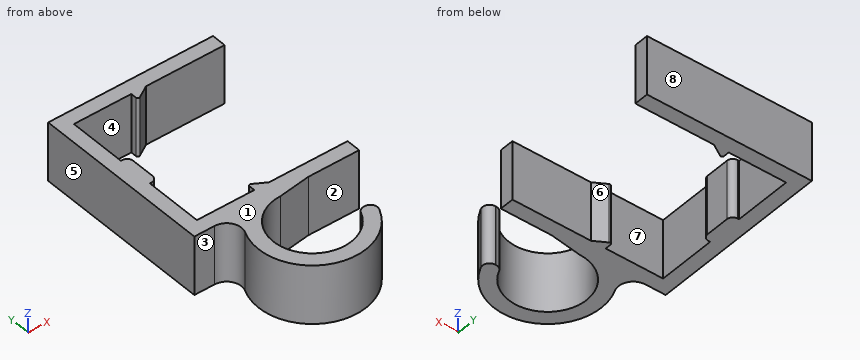
from build123d import *

# Parameters (mm, degrees)
F0_W     = 1.25
F0_H     = 6
F1_DEPTH = 10
F3_DEPTH = 10
F4_R     = 1.2
F5_R     = 2.5
F6_R     = 1
F7_R     = 0.3


with BuildPart() as f1:
    # F0 (on Top) → F1 (new body)
    with BuildSketch(Plane.XY):
        Polygon((0, -2.4), (0, 0), (-28, 0), (-28, -30.3), (0, -30.3), (0, -27.9), (-13.35, -27.9), (-15.85, -27.9), (-25.6, -27.9), (-25.6, -18.15), (-25.6, -12.15), (-25.6, -2.4), (-15.85, -2.4), (-13.35, -2.4), align=None)
        Polygon((-15.85, -3.9), (-13.35, -2.4), (-15.85, -2.4), align=None)
        Polygon((-15.85, -27.9), (-13.35, -27.9), (-15.85, -26.4), align=None)
        with Locations((-24.975, -15.15)):
            Rectangle(F0_W, F0_H)
    extrude(amount=F1_DEPTH)

    # F2 (on face) → F3 (join)
    with BuildSketch(Plane.XY.offset(10)):
        with BuildLine():
            ThreePointArc((-7.6731015896, -39.6488182922), (-19.3342450038, -41.6128057076), (-14, -31.0588802515))
            Line((-14, -31.0588802515), (-8.6386627198, -30.3))
            ThreePointArc((-8.6386627198, -30.3), (-22.5307966917, -40.9228820738), (-5.0890716816, -39.6488182922))
            Line((-5.0890716816, -39.6488182922), (-7.6731015896, -39.6488182922))
        make_face()
    extrude(amount=-F3_DEPTH)

    # F4
    f4_edges = [f1.edges().sort_by_distance(p)[0] for p in [
        (-7.673102, -39.648818, 5),
        (-5.089072, -39.648818, 5),
    ]]
    fillet(f4_edges, radius=F4_R)

    # F5
    f5_edges = [f1.edges().sort_by_distance(p)[0] for p in [
        (-19.361337, -30.3, 5),
    ]]
    fillet(f5_edges, radius=F5_R)

    # F6
    f6_edges = [f1.edges().sort_by_distance(p)[0] for p in [
        (-24.35, -12.15, 5),
        (-24.35, -18.15, 5),
    ]]
    fillet(f6_edges, radius=F6_R)

    # F7
    f7_edges = [f1.edges().sort_by_distance(p)[0] for p in [
        (-15.85, -3.9, 5),
        (-15.85, -26.4, 5),
    ]]
    fillet(f7_edges, radius=F7_R)


solid = f1.part
Check sheet for the modelled part. Datum: model origin and axes. Units: mm. Face numbers are marked on the shaded views. A direction names the side the tool comes from. Give positions to 0.01 mm unless a question says otherwise; leave off trailing zeros. Order: outer loops, then holes, each group sorted by start corner. A loop starts at its lowest first (then second) coordinate and runs counter-clockwise, first axis right, second up. Notation, with made-up numbers: M 67,23 L 84,23 A12 ccw 84,33 Z; hole C 88,20.5 d5. An arc over 180 degrees is marked long. Answer as CSV lines item,"result". Start each with the question number.
Item 1: Thickness scan on line 1 (Y direction, x = -14, z = 7.5); line 2 (Y direction, x = -14.75, z = 7.5); line 3 (X direction, y = -11.5, z = 6.75). Record the ranges inside material, lowest first. Write a range as [from, to].
Item 2: Tool access check on the marked faces 1, 2, 3, 4 and 5. Record the directions out of +Z, -Z, +X, -X, +Y, -Y that give a thin tool (end or side, any length) a straight path to the whole face; none if there is none.
Item 3: Mould release check, pull along X, two halves, no side actions. Record for the marked faces 6, 7 and 8: +X half, -X half, draft (parallel to the pull), parting line (faces both ways), or undercut.
Item 4: Cross-section at D-D on x = -18.5. Enter the section's corners in (y, z), plus the area to 3 significant figures.
Item 5: Cross-section at B-B on y = -43. Enter the section's corners in (x, z).
Item 6: Cross-section at A-A on x = -10. Enter the section's corners in (y, z).
Item 7: Gauge pin test, flat ends, axial feed: P1, Ø3, axis at y = -25, z = 5, coming from the +X side; P2, Ø5, axis at x = -20.5, z = 6.5, coming from the -Y side; P3, Ø2, axis at y = -16, z = 3, coming from the +X side. Record the tip position at first contact, or that the pin passes through.
Established:
1,line 1,"y = [-46.81, -44.31], [-31.06, -27.51], [-2.79, 0]"
1,line 2,"y = [-46.78, -44.27], [-31.1, -27.06], [-3.24, 0]"
1,line 3,"x = [-28, -25.6]"
2,face 1,"+Z, +X, -X, +Y, -Y"
2,face 2,"+Z, -Z, +X"
2,face 3,"+Z, -Z, -X, -Y"
2,face 4,"+Z, -Z"
2,face 5,"+Z, -Z, -X, +Y, -Y"
3,face 6,"+X half"
3,face 7,"undercut"
3,face 8,"draft"
4,outline,"M -45.62,0 L -42.55,0 L -42.55,10 L -45.62,10 Z; M -32.82,0 L -27.9,0 L -27.9,10 L -32.82,10 Z; M -2.4,0 L 0,0 L 0,10 L -2.4,10 Z"
4,area,"104 mm^2"
5,outline,"M -21.42,0 L -17.95,0 L -17.95,10 L -21.42,10 Z; M -10.05,0 L -6.58,0 L -6.58,10 L -10.05,10 Z"
6,outline,"M -45.89,0 L -42.97,0 L -42.97,10 L -45.89,10 Z; M -30.49,0 L -27.9,0 L -27.9,10 L -30.49,10 Z; M -2.4,0 L 0,0 L 0,10 L -2.4,10 Z"
7,P1,"stops at x = -25.6"
7,P2,"stops at y = -45.89"
7,P3,"stops at x = -24.35"
